Source: CAD feature listing. Evaluate the final solid. Frame: model axes, mm. Coordinates: 2 decimals unless noted, no trailing zeros. Write each loop counter-clockwise with the first axis right and the second up, starting at its lowest first coordinate (ties: lowest second). Pieces come first, ordered by that corner, then holes. Notation, with made-up numbers: M 80,17 L 84,17 A17 cw 84,28 Z; hole C -13.75,-6.75 d9. An arc over 180 degrees is marked long. Write item = value, one per line. Start each with the question number.
1. Pin query (flat end, axial travel): pin 1 Ø23 at (x, y) = (0, 0) entering from +Z; pin 2 Ø1 at (x, z) = (30, 2) entering from -Y; pin 3 Ø1.5 at (y, z) = (-9, 2) entering from -X. Return the tip coordinate at first contact, or that it passes through.
2. Pull-direction query (X, two-part tool) for faces 1 (the face through (0, -19, 2)), 2 (the face through (-15.46, 3, -0.06)); classes: pulls with the +X half, pulls with the -X half, needs draft (parallel to the pull), parting line crosses it, or undercut.
3. Section query A-A (y = 0). Output: boundary loops of the cut face in (x, z).
4. Section query C-C (z = 0.25). Output: boundary loops of the cut face in (x, y), then the cut area to 3 significant figures.
5. Line query: line 1 along Y through (x, z) = (23.5, -2.25); line 2 along Y through (x, z) = (29, 0); line 3 along X through (y, z) = (7, 2.25). Output: solid intervals per line, ascending.
6. Section query B-B (x = -3.5). Output: boundary loops of the cut face in (y, z), then the cut area to 3 significant figures.
7. Section query D-D (y = 8). Give the number of separate pieces and of enclosed holes in the cut face, then the cut area to 3 significant figures.
```python
from build123d import *

# Parameters (mm, degrees)
F0_R        = 10
F1_DEPTH    = 4
F2_R        = 5
F3_T1_DEPTH = 50
F3_T4_ANGLE = 180
F3_T6_ANGLE = 180


# Not quite as in the source:
# - a fillet or chamfer that OpenCascade refuses, or shapes differently, is made with other operations: its cross-section is extruded or revolved along the edge and cut away or added


with BuildPart() as f1:
    # F0 (on Top) → F1 (new body, symmetric)
    with BuildSketch(Plane.XY):
        with BuildLine():
            Line((25, 20), (-25, 20))
            ThreePointArc((-25, 20), (-45, 0), (-25, -20))
            Line((-25, -20), (25, -20))
            ThreePointArc((25, -20), (45, 0), (25, 20))
        make_face()
        with Locations((-25, 0)):
            Circle(F0_R, mode=Mode.SUBTRACT)
        Circle(F0_R, mode=Mode.SUBTRACT)
        with Locations((25, 0)):
            Circle(F0_R, mode=Mode.SUBTRACT)
    extrude(amount=F1_DEPTH, both=True)

    # F2
    f2_edges = [f1.edges().sort_by_distance(p)[0] for p in [
        (0, 20, 4),
        (-45, 0, 4),
        (0, -20, 4),
        (45, 0, 4),
    ]]
    fillet(f2_edges, radius=F2_R)

    # F3: fillet of radius 5 on 4 edges, made by hand

    # F3_s2 → F3_t1 (cut)
    with BuildSketch(Plane.YZ.offset(-25)):
        with BuildLine():
            ThreePointArc((-15.417424305, -4), (-18.1560370926, -3.1833001327), (-20, -1))
            Line((-20, -1), (-20, -4))
            Line((-20, -4), (-15.417424305, -4))
        make_face()
        with BuildLine():
            ThreePointArc((20, -1), (18.1560370926, -3.1833001327), (15.417424305, -4))
            Line((15.417424305, -4), (20, -4))
            Line((20, -4), (20, -1))
        make_face()
    extrude(amount=F3_T1_DEPTH, mode=Mode.SUBTRACT)

    # F3_s3 → F3_t4 (revolve, cut)
    with BuildSketch(Plane.YZ.offset(25)):
        with BuildLine():
            ThreePointArc((-20, -1), (-18.1560370926, -3.1833001327), (-15.417424305, -4))
            Line((-15.417424305, -4), (-20, -4))
            Line((-20, -4), (-20, -1))
        make_face()
    revolve(axis=Axis((25, 0, -4), (0, 0, 1)), revolution_arc=F3_T4_ANGLE, mode=Mode.SUBTRACT)

    # F3_s5 → F3_t6 (revolve, cut)
    with BuildSketch(Plane.YZ.offset(-25)):
        with BuildLine():
            ThreePointArc((15.417424305, -4), (18.1560370926, -3.1833001327), (20, -1))
            Line((20, -1), (20, -4))
            Line((20, -4), (15.417424305, -4))
        make_face()
    revolve(axis=Axis((-25, 0, -4), (0, 0, 1)), revolution_arc=F3_T6_ANGLE, mode=Mode.SUBTRACT)


solid = f1.part
```
Results are:
q1.pin_1 = 4
q1.pin_2 = -18.7
q1.pin_3 = -42.4
q2.face_1 = needs draft
q2.face_2 = undercut
q3.outline = M -45,-1 A5 ccw -40.42,-4 L -35,-4 L -35,4 L -40,4 A5 ccw Z; M -15,-4 L -10,-4 L -10,4 L -15,4 Z; M 10,-4 L 15,-4 L 15,4 L 10,4 Z; M 35,-4 L 40.42,-4 A5 ccw 45,-1 A5 ccw 40,4 L 35,4 Z
q4.outline = M -25,-19.84 L 25,-19.84 A19.84 ccw 25,19.84 L -25,19.84 A19.84 ccw Z; hole C -25,0 d20; hole C 0,0 d20; hole C 25,0 d20
q4.area = 2,280 mm^2
q5.line_1 = -19.22 to -9.89, 9.89 to 19.22
q5.line_2 = -19.49 to -9.17, 9.17 to 19.49
q5.line_3 = -42.45 to -32.14, -17.86 to -7.14, 7.14 to 17.86, 32.14 to 42.45
q6.outline = M -20,-1 A5 ccw -15.42,-4 L -9.37,-4 L -9.37,4 L -15,4 A5 ccw Z; M 9.37,-4 L 15.42,-4 A5 ccw 20,-1 A5 ccw 15,4 L 9.37,4 Z
q6.area = 152 mm^2
q7.separate_pieces = 4
q7.enclosed_holes = 0
q7.area = 385 mm^2
